Autodesk Inventor part; units mm, degrees
ref_plane "YZ Plane" through (0, 0, 0) normal (1, 0, 0) x (0, 1, 0)
ref_plane "XZ Plane" through (0, 0, 0) normal (0, 1, 0) x (-1, 0, 0)
ref_plane "XY Plane" through (0, 0, 0) normal (0, 0, 1) x (1, 0, 0)
sketch "Sketch2" plane through (0, 0, 0) normal (0, 0, 1) x (1, 0, 0)
  line L0 (0, 0) -> (5, 0)
  line L1 (5, 0) -> (5, 5)
  line L2 (5, 5) -> (0, 5)
  line L3 (0, 5) -> (0, 0)
  line L4 (0, 5) -> (65, 5)
  line L5 (65, 5) -> (65, 30)
  line L6 (65, 30) -> (0, 30)
  line L7 (0, 30) -> (0, 5)
  line L8 (10, 0) -> (15, 0)
  line L9 (15, 0) -> (15, 5)
  line L10 (10, 5) -> (10, 0)
  line L11 (20, 0) -> (25, 0)
  line L12 (25, 0) -> (25, 5)
  line L13 (20, 5) -> (20, 0)
  line L14 (30, 0) -> (35, 0)
  line L15 (35, 0) -> (35, 5)
  line L16 (30, 5) -> (30, 0)
  line L17 (40, 0) -> (45, 0)
  line L18 (45, 0) -> (45, 5)
  line L19 (40, 5) -> (40, 0)
  line L20 (50, 0) -> (55, 0)
  line L21 (55, 0) -> (55, 5)
  line L22 (50, 5) -> (50, 0)
  line L23 (60, 0) -> (65, 0)
  line L24 (65, 0) -> (65, 5)
  line L25 (60, 5) -> (60, 0)
  line L26 (65, 25) -> (70, 25)
  line L27 (70, 25) -> (70, 20)
  line L28 (70, 20) -> (65, 20)
  line L29 (65, 20) -> (65, 25)
  line L30 (65, 15) -> (70, 15)
  line L31 (70, 15) -> (70, 10)
  line L32 (70, 10) -> (65, 10)
  line L33 (65, 10) -> (65, 15)
  line L34 (0, 35) -> (5, 35)
  line L35 (5, 35) -> (5, 30)
  line L36 (5, 30) -> (0, 30)
  line L37 (0, 30) -> (0, 35)
  line L38 (15, 35) -> (15, 30)
  line L39 (15, 30) -> (10, 30)
  line L40 (10, 35) -> (15, 35)
  line L41 (10, 30) -> (10, 35)
  line L42 (25, 35) -> (25, 30)
  line L43 (25, 30) -> (20, 30)
  line L44 (20, 35) -> (25, 35)
  line L45 (20, 30) -> (20, 35)
  line L46 (35, 35) -> (35, 30)
  line L47 (35, 30) -> (30, 30)
  line L48 (30, 35) -> (35, 35)
  line L49 (30, 30) -> (30, 35)
  line L50 (45, 35) -> (45, 30)
  line L51 (45, 30) -> (40, 30)
  line L52 (40, 35) -> (45, 35)
  line L53 (40, 30) -> (40, 35)
  line L54 (55, 35) -> (55, 30)
  line L55 (55, 30) -> (50, 30)
  line L56 (50, 35) -> (55, 35)
  line L57 (50, 30) -> (50, 35)
  line L58 (65, 35) -> (65, 30)
  line L59 (65, 30) -> (60, 30)
  line L60 (60, 35) -> (65, 35)
  line L61 (60, 30) -> (60, 35)
  line L62 (-5, 35) -> (0, 35)
  line L63 (0, 35) -> (0, 0)
  line L64 (0, 0) -> (-5, 0)
  line L65 (-5, 0) -> (-5, 35)
  line L66 (-5, 5) -> (0, 5)
  line L67 (0, 5) -> (0, 0)
  line L68 (0, 0) -> (-5, 0)
  line L69 (-5, 0) -> (-5, 5)
  line L70 (55, 35) -> (60, 35)
  line L71 (60, 35) -> (60, 30)
  line L72 (60, 30) -> (55, 30)
  line L73 (55, 30) -> (55, 35)
  line L74 (60, 25) -> (65, 25)
  line L75 (65, 25) -> (65, 20)
  line L76 (65, 20) -> (60, 20)
  line L77 (60, 20) -> (60, 25)
  line L78 (60, 15) -> (65, 15)
  line L79 (65, 15) -> (65, 10)
  line L80 (65, 10) -> (60, 10)
  line L81 (60, 10) -> (60, 15)
  line L82 (60, 30) -> (65, 30)
  line L83 (65, 30) -> (65, 5)
  line L84 (65, 5) -> (60, 5)
  line L85 (60, 5) -> (60, 30)
  dimension "d97" = 10
  dimension "d102" = 25
  dimension "d105" = 10
extrude "Extrusion3" add sketch "Sketch2" along normal blind 5 contours L3 L2 L1 L0 | L7 L6 L85 L77 L81 L4 L2 | L66 L65 L62 L37 L7 | L37 L34 L35 L6 | L4 L9 L8 L10 | L41 L40 L38 L6 | L4 L12 L11 L13 | L45 L44 L42 L6 | L4 L15 L14 L16 | L49 L48 L46 L6 | L4 L18 L17 L19 | L53 L52 L50 L6 | L4 L21 L20 L22 | L57 L56 L54 L6 | L85 L80 L5 L4 | L4 L24 L23 L25 | L54 L70 L61 L6 | L6 L5 L74 L85 | L85 L76 L5 L78
properties part number "backside"
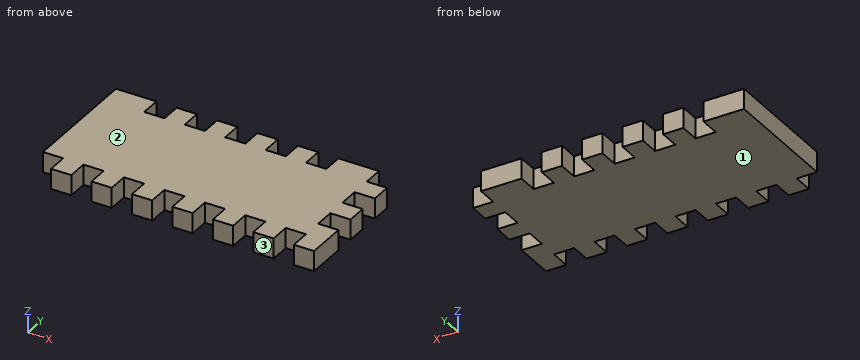
Geometry: final body of the model. Coordinates: model frame, mm. Face numbers are marked on the shaded views. Coordinates: 2 decimals unless noted, no trailing zeros. Loops run counter-clockwise (first coordinate to the right, second up) from the corner with the lowest first, then second, coordinate; pieces in that order, holes last. Notation, with made-up numbers: M 77,-15.75 L 127,-15.75 A18 ccw 127,-7.75 Z; hole C 42.25,61.25 d3. An arc over 180 degrees is marked long. Put each result on its own line as item: value.
(1) Cut plane C-C on y = 12.5. Return the cut outline in (x, z), then the cut area to 3 significant figures.
Answer sheet:
outline: M -5,0 L 60,0 L 60,5 L -5,5 Z
area: 325 mm^2
(2) Cut plane B-B on x = 26.5. Return the cut outline in (y, z), then the cut area to 3 significant figures.
Answer sheet:
outline: M 5,0 L 30,0 L 30,5 L 5,5 Z
area: 125 mm^2
(3) Cut plane A-A on y = 31.5. Return the cut outline in (x, z).
Answer sheet:
outline: M -5,0 L 5,0 L 5,5 L -5,5 Z; M 10,0 L 15,0 L 15,5 L 10,5 Z; M 20,0 L 25,0 L 25,5 L 20,5 Z; M 30,0 L 35,0 L 35,5 L 30,5 Z; M 40,0 L 45,0 L 45,5 L 40,5 Z; M 50,0 L 60,0 L 60,5 L 50,5 Z
(4) Material intervals for probe 1 along Y at (x, z) = (61, 4.85); probe 2 along Y at (x, z) = (19, 2.3); probe 3 along X at (y, z) = (12, 4), sorted ascending.
Answer sheet:
probe 1: y = 0 to 10, 15 to 20, 25 to 30
probe 2: y = 5 to 30
probe 3: x = -5 to 60
(5) First-contact query: pin 1 (2.5 mm diameter, centred on x = 57, z = 3, fed in from -Y); pin 2 (2.5 mm diameter, centred on x = 17.5, z = 3, fed in from +Y); pin 3 (2.5 mm diameter, centred on y = 12, z = 2.5, fed in from +X); pin 4 (10 mm diameter, centred on x = 56.5, y = 13, fed in from -Z). Flat tips, straight axial feed; report the tip coordinate or a pass-through.
Answer sheet:
pin 1: stops at y = 5
pin 2: stops at y = 30
pin 3: stops at x = 60
pin 4: stops at z = 0
(6) Draft query along Z for the marked faces 1, 2 and 3. Return one class per face: pulls with the +Z half, pulls with the -Z half, needs draft (parallel to the pull), parting line crosses it, or undercut.
Answer sheet:
face 1: pulls with the -Z half
face 2: pulls with the +Z half
face 3: needs draft
